Autodesk Inventor part; units mm, degrees
ref_plane "YZ Plane" through (0, 0, 0) normal (1, 0, 0) x (0, 1, 0)
ref_plane "XZ Plane" through (0, 0, 0) normal (0, 1, 0) x (-1, 0, 0)
ref_plane "XY Plane" through (0, 0, 0) normal (0, 0, 1) x (1, 0, 0)
sketch "Sketch1" plane through (0, 0, 0) normal (0, 1, 0) x (-1, 0, 0)
  line L0 (0, -4.766) -> (-4.1275, -2.383)
  line L1 (-4.1275, -2.383) -> (-4.1275, 2.383)
  line L2 (-4.1275, 2.383) -> (0, 4.766)
  line L3 (0, 4.766) -> (4.1275, 2.383)
  line L4 (4.1275, 2.383) -> (4.1275, -2.383)
  line L5 (4.1275, -2.383) -> (0, -4.766)
  point P0 (0, 0)
  point P1 (0, 0)
  dimension "d0" = 8.255
extrude "Extrusion1" add sketch "Sketch1" along normal blind 38.1
sketch "Sketch2" plane through (0, 38.1, 0) normal (0, 1, 0) x (1, 0, 0)
  circle A0 centre (0, 0) radius 9.2075
  dimension "d3" = 18.415
extrude "Extrusion2" add sketch "Sketch2" along normal blind 47.625
sketch "Sketch3" plane through (0, 85.725, 0) normal (0, 1, 0) x (1, 0, 0)
  line L0 (-1.8415, 1.8415) -> (1.8415, 1.8415)
  line L1 (1.8415, 1.8415) -> (1.8415, -1.8415)
  line L2 (1.8415, -1.8415) -> (-1.8415, -1.8415)
  line L3 (-1.8415, -1.8415) -> (-1.8415, 1.8415)
  point P0 (0, 0)
  point P1 (0, 0)
  dimension "d6" = 3.683
extrude "Extrusion3" add sketch "Sketch3" along normal blind 50.8
Could you check a few things on this model? Use its own coordinates, in mm. A direction names the side the tool comes from. Coordinates: 2 decimals unless noted, no trailing zeros. Write each loop counter-clockwise with the first axis right and the second up, starting at its lowest first coordinate (ties: lowest second). Pieces come first, ordered by that corner, then holes. Notation, with made-up numbers: M 36.5,0.25 L 90.5,0.25 A12 ccw 90.5,6.25 Z; hole C -30,-17.5 d11. An arc over 180 degrees is marked long. Answer as CSV lines item,"result". Start each with the question number.
1) I want a section at C-C, the plane y = 91.5. Please give me the cut outline in (x, z).
2) I want a section at A-A, the plane z = 0. Please give me the cut outline in (x, y) (1 decimal).
3) I want a section at B-B, the plane y = 23. Please give me the cut outline in (x, z), and give its area (3 significant figures).
4) I want a section at D-D, the plane x = 6. Please give me the cut outline in (y, z) (3 decimals), and give its area (3 significant figures).
5) For P1, Ø3, axis at x = -4.5, z = -4, coming from the -Y side; P2, Ø1.4, axis at y = 16.5, z = 0.5, coming from the -X side; P3, Ø1.4, axis at y = 14.5, z = -1, coming from the +X side; P4, Ø5, axis at y = 93, z = 5, coming from the -X side, each with a flat end and sliding along its axis, tell me the tip position at first contact or that it passes through.
6) For faces 1 (the flat face through (4.128, 19, 0)), 2 (the flat face through (0, 111, 1.842)), 3 (the flat face through (-1.842, 111, 0)), 4 (the flat face through (-4.128, 19, 0)), 5 (the flat face through (1.842, 111, 0)), which set-ups out of +Z, -Z, +X, -X, +Y, -Y let a thin tool reach every point of the face, with its end or its side?
7) Please list where these lines run through material, in increasing order: line 1 (Y direction, x = -4.25, z = -5.25) (3 decimals); line 2 (Z direction, x = 0.75, y = 97). Write a range as from..to.
Data:
1,outline,"M -1.84,-1.84 L 1.84,-1.84 L 1.84,1.84 L -1.84,1.84 Z"
2,outline,"M -9.2,38.1 L -4.1,38.1 L -4.1,0 L 4.1,0 L 4.1,38.1 L 9.2,38.1 L 9.2,85.7 L 1.8,85.7 L 1.8,136.5 L -1.8,136.5 L -1.8,85.7 L -9.2,85.7 Z"
3,outline,"M -4.13,-2.38 L 0,-4.77 L 4.13,-2.38 L 4.13,2.38 L 0,4.77 L -4.13,2.38 Z"
3,area,"59.0 mm^2"
4,outline,"M 38.1,-6.984 L 85.725,-6.984 L 85.725,6.984 L 38.1,6.984 Z"
4,area,"665 mm^2"
5,P1,"stops at y = 38.1"
5,P2,"stops at x = -4.13"
5,P3,"stops at x = 4.13"
5,P4,"passes through"
6,face 1,"+Z, -Z, +X, -Y"
6,face 2,"+Z, +X, -X, +Y"
6,face 3,"+Z, -Z, -X, +Y"
6,face 4,"+Z, -Z, -X, -Y"
6,face 5,"+Z, -Z, +X, +Y"
7,line 1,"y = 38.1..85.725"
7,line 2,"z = -1.84..1.84"
